Could you check a few things on this drawing? It's one solid part, dimensions in mm from its lowest x, y, z. A direction names the side the tool comes from. Round coordinates to 2 decimals unless told otherwise and drop trailing zeros. Order: outer loops, then holes, each group sorted by start corner. A loop starts at its lowest first (then second) coordinate and runs counter-clockwise, first axis right, second up. Notation, with made-up numbers: (68, 33) -> (121, 33) arc R22 ccw to (121, 67) -> close; hole circle Ø10 at (-37, 89). An arc over 180 degrees is marked (long way). Use a Markdown table: item, result. Add a question column.
(1) If I drill on probe 1 along X at (y, z) = (12.7, 64) (1 decimal); probe 2 along Z at (x, y) = (36, 24.25) (1 decimal); probe 3 along X at (y, z) = (15.25, 41), over which ranges is the centre line in solid material (lowest first)?
(2) On a 3-axis mill with a long thin cutter (end or side, diameter ignored), from which of +Z, -Z, +X, -X, +Y, -Y can I reach the whole of each face in a straight line? I mean the marked faces 1 and 2. Say none if no direction works.
(3) I want a section at A-A, the plane x = 67. Please give me the cut outline in (y, z) (1 decimal).
(4) I'm going to push a flat-ended pin straight in: P1, Ø1, axis at x = 22, z = 8.5, coming from the -Y side. Where does the tip first touch, or does it pass through?
(5) Thinking about a two-plate mould opening in Z: for the marked faces 3, 4, 5 and 6, which applies, pulls with the +Z half, pulls with the -Z half, needs draft (parallel to the pull), parting line crosses it, or undercut?
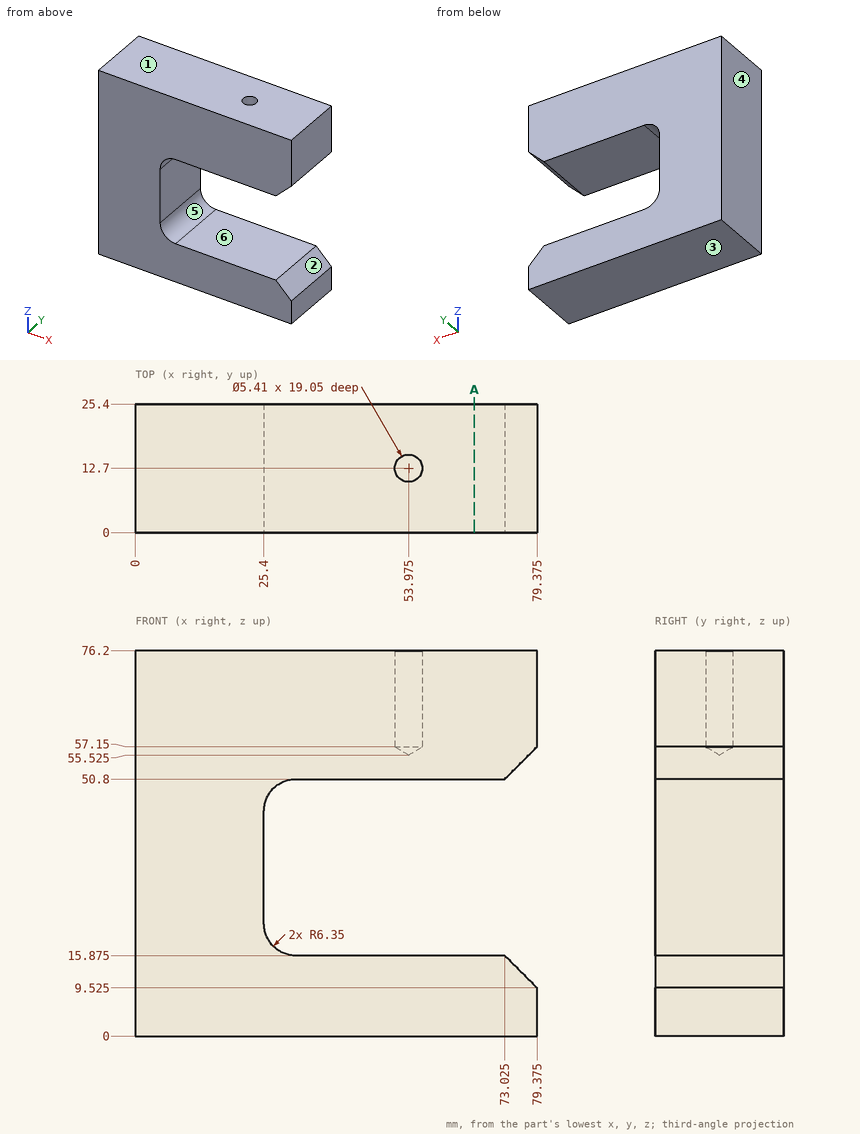
Taken from the geometry:
| question | item | result |
|---|---|---|
| 1 | probe 1 | x = 0 to 51.3, 56.7 to 79.4 |
| 1 | probe 2 | z = 0 to 15.9, 50.8 to 76.2 |
| 1 | probe 3 | x = 0 to 25.4 |
| 2 | face 1 | +Z, +X, -X, +Y, -Y |
| 2 | face 2 | +X, +Y, -Y |
| 3 | outline | (0, 0) -> (25.4, 0) -> (25.4, 15.9) -> (0, 15.9) -> close; (0, 50.8) -> (25.4, 50.8) -> (25.4, 76.2) -> (0, 76.2) -> close |
| 4 | P1 | stops at y = 0 |
| 5 | face 3 | pulls with the -Z half |
| 5 | face 4 | needs draft |
| 5 | face 5 | undercut |
| 5 | face 6 | undercut |
